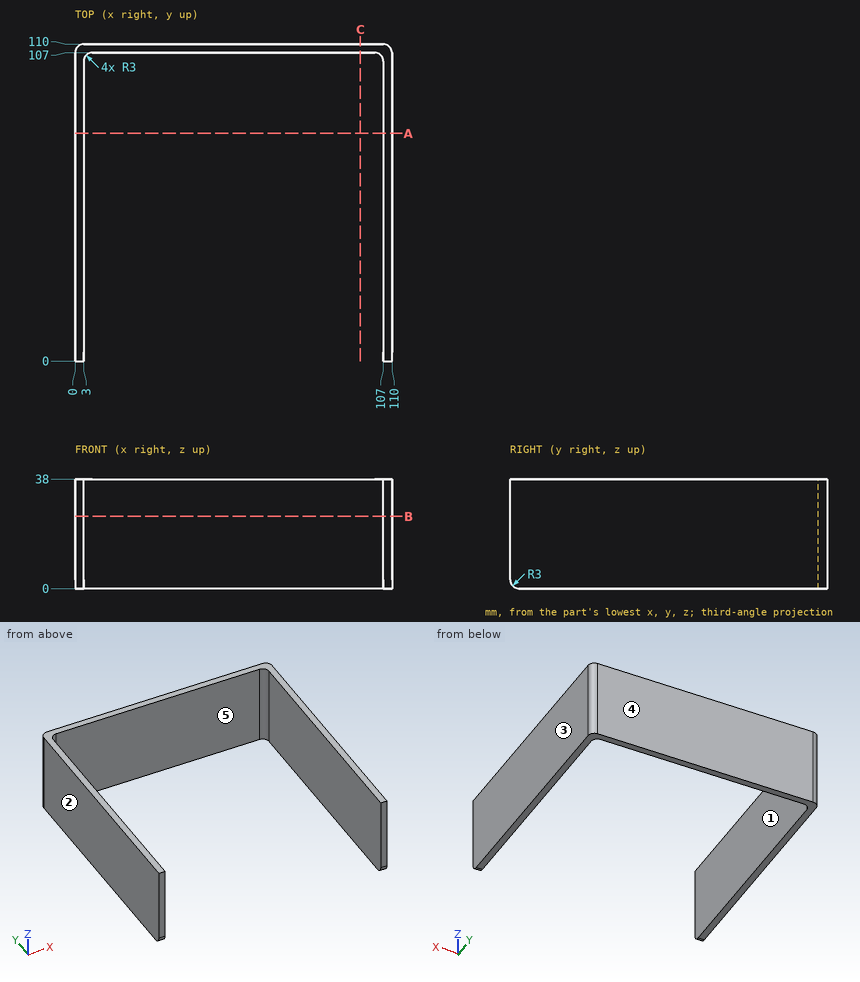
Input: dimensioned drawing with shaded views. Units: mm. Origin: part minimum x, y, z. A direction names the side the tool comes from. Round coordinates to 2 decimals unless told otherwise and drop trailing zeros. Order: outer loops, then holes, each group sorted by start corner. A loop starts at its lowest first (then second) coordinate and runs counter-clockwise, first axis right, second up.
1. Cut plane C-C, the plane x = 99. Output: boundary loops of the cut face in (y, z), then the cut area to 3 significant figures.
The answers:
outline: (107, 0) - (110, 0) - (110, 38) - (107, 38) - close
area: 114 mm2
2. Mould query, pull axis X, two halves, no side actions, for the marked faces 3, 4 and 5. Classes: released by +X, released by -X, zero draft, split by the parting line, or undercut.
The answers:
face 3: released by +X
face 4: zero draft
face 5: undercut
3. Set-up query: the marked faces 1 and 2. Return all of +Z, -Z, +X, -X, +Y, -Y with unobstructed straight access to the full face (end or side cutting, diameter ignored); none if empty.
The answers:
face 1: +Z, -Z, -Y
face 2: +Z, -Z, -X, +Y, -Y
4. Cut plane A-A, the plane y = 79. Output: boundary loops of the cut face in (x, z).
The answers:
outline: (0, 0) - (3, 0) - (3, 38) - (0, 38) - close; (107, 0) - (110, 0) - (110, 38) - (107, 38) - close
5. Pin query (flat end, axial travel): P1, Ø8, axis at y = 67, z = 7.5, coming from the -X side; P2, Ø2, axis at x = 31.5, z = 19.5, coming from the -Y side. Return the tip coordinate at first contact, or that it passes through.
The answers:
P1: stops at x = 0
P2: stops at y = 107
6. Material intervals for line 1 (X direction, y = 61.5, z = 31); line 2 (Y direction, x = 18.5, z = 25.5); line 3 (X direction, y = 106, z = 16.5), sorted ascending.
The answers:
line 1: x = 0 to 3, 107 to 110
line 2: y = 107 to 110
line 3: x = 0 to 3.76, 106.24 to 110
7. Cut plane B-B, the plane z = 25. Output: boundary loops of the cut face in (x, y).
The answers:
outline: (0, 0) - (3, 0) - (3, 104) arc R3 cw to (6, 107) - (104, 107) arc R3 cw to (107, 104) - (107, 0) - (110, 0) - (110, 107) arc R3 ccw to (107, 110) - (3, 110) arc R3 ccw to (0, 107) - close
